from build123d import *
from OCP.BRepFilletAPI import BRepFilletAPI_MakeChamfer

# Parameters (mm, degrees)
BOSS_EXTRUDE1_DEPTH = 12
BOSS_EXTRUDE2_DEPTH = 50
BOSS_EXTRUDE3_DEPTH = 12
SKETCH4_R           = 120
BOSS_EXTRUDE4_DEPTH = 500
SKETCH5_R           = 172.646944325
BOSS_EXTRUDE5_DEPTH = 12
CHAMFER1_SIZE       = 56.712818196
CHAMFER1_SIZE_2     = 10
SKETCH6_R           = 120
BOSS_EXTRUDE6_DEPTH = 330
SKETCH8_R           = 172.646944325
BOSS_EXTRUDE7_DEPTH = 12
CHAMFER2_SIZE       = 6
CHAMFER2_SIZE2      = 16.484864517
SKETCH9_W           = 370
SKETCH9_H           = 370
BOSS_EXTRUDE8_DEPTH = 370
SKETCH10_R          = 100
CUT_EXTRUDE1_DEPTH  = 900
CHAMFER3_SIZE       = 30
CHAMFER3_SIZE2      = 51.961524227


with BuildPart() as part:
    # Sketch1 → Boss-Extrude1 (new body)
    with BuildSketch(Plane.XY):
        Polygon((202.072594216, 0), (101.036297108, 175), (-101.036297108, 175), (-202.072594216, 0), (-101.036297108, -175), (101.036297108, -175), align=None)
    extrude(amount=BOSS_EXTRUDE1_DEPTH)

    # Sketch2 → Boss-Extrude2 (add)
    with BuildSketch(Plane.XY.offset(12)):
        Polygon((147.887498821, 0), (73.943749411, 128.074330881), (-73.943749411, 128.074330881), (-147.887498821, 0), (-73.943749411, -128.074330881), (73.943749411, -128.074330881), align=None)
    extrude(amount=BOSS_EXTRUDE2_DEPTH)

    # Sketch3 → Boss-Extrude3 (add)
    with BuildSketch(Plane.XY.offset(62)):
        Polygon((202.072594216, 0), (101.036297108, 175), (-101.036297108, 175), (-202.072594216, 0), (-101.036297108, -175), (101.036297108, -175), align=None)
    extrude(amount=BOSS_EXTRUDE3_DEPTH)

    # Sketch4 → Boss-Extrude4 (add)
    with BuildSketch(Plane.XY.offset(74)):
        Circle(SKETCH4_R)
    extrude(amount=BOSS_EXTRUDE4_DEPTH)

    # Sketch5 → Boss-Extrude5 (add)
    with BuildSketch(Plane.XY.offset(574)):
        Circle(SKETCH5_R)
    extrude(amount=BOSS_EXTRUDE5_DEPTH)

    # Chamfer1
    # the kernel refuses this chamfer: 56.712818196, 10 mm, written as the material it adds along each edge
    with BuildSketch(Plane(origin=(0, 0, 574), x_dir=(1, 0, 0), z_dir=(0, -1, 0))) as chamfer1_piece_1_section:
        Polygon((120 + CHAMFER1_SIZE, 0), (120, -CHAMFER1_SIZE_2), (120, 0), align=None)
    chamfer1_piece_1 = revolve(axis=Axis((0, 0, 574), (0, 0, 1)), mode=Mode.PRIVATE)
    chamfer1_piece_1 = chamfer1_piece_1 & Plane(origin=(0, 0, 569.114385433), x_dir=(1, 0, 0), z_dir=(0, 0, -1)) * Cylinder(172.646944325, 707, mode=Mode.PRIVATE)
    add(chamfer1_piece_1)

    # Sketch6 → Boss-Extrude6 (add)
    with BuildSketch(Plane.XY.offset(586)):
        Circle(SKETCH6_R)
    extrude(amount=BOSS_EXTRUDE6_DEPTH)

    # Sketch8 → Boss-Extrude7 (add)
    with BuildSketch(Plane.XY.offset(916)):
        Circle(SKETCH8_R)
    extrude(amount=BOSS_EXTRUDE7_DEPTH)

    # Chamfer2
    chamfer2_edges = [part.edges().sort_by_distance(p)[0] for p in [
        (-120, 0, 916),
    ]]
    chamfer2_side = [part.faces().sort_by_distance(p)[0] for p in [
        (-120, 0, 751),
    ]]
    chamfer(chamfer2_edges, length=CHAMFER2_SIZE, length2=CHAMFER2_SIZE2, reference=chamfer2_side[0])

    # Sketch9 → Boss-Extrude8 (add)
    with BuildSketch(Plane.XY.offset(928)):
        Rectangle(SKETCH9_W, SKETCH9_H)
    extrude(amount=BOSS_EXTRUDE8_DEPTH)

    # Sketch10 → Cut-Extrude1 (cut)
    with BuildSketch(Plane.XY.offset(1298)):
        Circle(SKETCH10_R)
    extrude(amount=-CUT_EXTRUDE1_DEPTH, mode=Mode.SUBTRACT)

    # Chamfer3: one chamfer whose edges measure the first distance from different faces: ONE call of the kernel's chamfer builder (chamfer() names one face for all edges)
    chamfer3_edges_1 = [part.edges().sort_by_distance(p)[0] for p in [
        (185, 0, 1298),
    ]]
    chamfer3_side_1 = [part.faces().sort_by_distance(p)[0] for p in [
        (185, 0, 1113),
    ]]
    chamfer3_edges_2 = [part.edges().sort_by_distance(p)[0] for p in [
        (0, 185, 1298),
    ]]
    chamfer3_side_2 = [part.faces().sort_by_distance(p)[0] for p in [
        (0, 185, 1113),
    ]]
    chamfer3_edges_3 = [part.edges().sort_by_distance(p)[0] for p in [
        (-185, 0, 1298),
    ]]
    chamfer3_side_3 = [part.faces().sort_by_distance(p)[0] for p in [
        (-185, 0, 1113),
    ]]
    chamfer3_edges_4 = [part.edges().sort_by_distance(p)[0] for p in [
        (0, -185, 1298),
    ]]
    chamfer3_side_4 = [part.faces().sort_by_distance(p)[0] for p in [
        (0, -185, 1113),
    ]]
    chamfer3 = BRepFilletAPI_MakeChamfer(part.part.solid().wrapped)
    for e in chamfer3_edges_1:
        chamfer3.Add(CHAMFER3_SIZE, CHAMFER3_SIZE2, e.wrapped, chamfer3_side_1[0].wrapped)  # the first distance lies on this face
    for e in chamfer3_edges_2:
        chamfer3.Add(CHAMFER3_SIZE, CHAMFER3_SIZE2, e.wrapped, chamfer3_side_2[0].wrapped)  # the first distance lies on this face
    for e in chamfer3_edges_3:
        chamfer3.Add(CHAMFER3_SIZE, CHAMFER3_SIZE2, e.wrapped, chamfer3_side_3[0].wrapped)  # the first distance lies on this face
    for e in chamfer3_edges_4:
        chamfer3.Add(CHAMFER3_SIZE, CHAMFER3_SIZE2, e.wrapped, chamfer3_side_4[0].wrapped)  # the first distance lies on this face
    add(Compound.cast(chamfer3.Shape()), mode=Mode.REPLACE)


solid = part.part
Design review of the part built by this model. Coordinates are the model's own, in mm. A direction names the side the tool comes from. Coordinates: 2 decimals unless noted, no trailing zeros. Write each loop counter-clockwise with the first axis right and the second up, starting at its lowest first coordinate (ties: lowest second). Pieces come first, ordered by that corner, then holes. Notation, with made-up numbers: (-12.75, -7) - (41.25, -7) arc R29 cw to (41.25, 32) - close; hole circle Ø2 at (-12.75, -38.5). An arc over 180 degrees is marked (long way). One line per item, written item: value.
1) Add section B-B (z = 200). State the section outline as (x, y) points.
Answer sheet:
outline: circle Ø240 at (0, 0)
2) Insertion check: pin 1 (3 mm diameter, centred on x = 38, z = 288, fed in from +Y); pin 2 (6 mm diameter, centred on x = -29, z = 268, fed in from -Y); pin 3 (12 mm diameter, centred on y = -12, z = 574, fed in from +X). Each pin has a flat end and moves straight along its axis. Give the tip position at first contact, or say it passes through.
Answer sheet:
pin 1: stops at y = 114.31
pin 2: stops at y = -117.15
pin 3: stops at x = 172.54
3) For faces 4 (the face through (150.85, -88.72, 67.92)), 5 (the face through (-110.4, 64.93, 36.65)), 6 (the face through (104, 79, 62)), 7 (the face through (-150.85, 88.72, 67.92)), list the 3-axis set-ups (+Z, -Z, +X, -X, +Y, -Y) from which the entire face can be reached by the end or side of a thin tool; tool diameter is ignored.
Answer sheet:
face 4: -Z, +X, -Y
face 5: -X, +Y
face 6: none
face 7: -Z, -X, +Y
4) Mouldability with a two-part tool opening along Z and no side actions: class faces 1 (the face through (111.433, 63.141, 36.65)), 2 (the face through (158.656, -2.59, 1283.21)), 3 (the face through (185, -3, 1096)) as +Z half, -Z half, draft (parallel to the pull), parting line (faces both ways), or undercut.
Answer sheet:
face 1: undercut
face 2: +Z half
face 3: draft
5) To check wall thickness, follow probe 1 along Y at (x, z) = (0, 1105); probe 2 along Z at (x, y) = (56, -124); probe 3 along Z at (x, y) = (169, 35). State the ranges of each line that lie inside material, in increasing order.
Answer sheet:
probe 1: y = -185 to -100, 100 to 185
probe 2: z = 0 to 74, 566.83 to 586, 915.84 to 1298
probe 3: z = 0 to 12, 62 to 74, 573.27 to 586, 916 to 1277.24
6) Add section A-A (z = 492). State the section outline as (x, y) points.
Answer sheet:
outline: circle Ø240 at (0, 0); hole circle Ø200 at (0, 0)
7) Add section C-C (z = 1002). State the section outline as (x, y) points, plus the area to 3 significant figures.
Answer sheet:
outline: (-185, -185) - (185, -185) - (185, 185) - (-185, 185) - close; hole circle Ø200 at (0, 0)
area: 105,000 mm2
